Can you work these out from the model? Positions are in its coordinate system, mm. Round coordinates to 2 decimals unless told otherwise and drop trailing zeros. Order: outer loops, then holes, each group sorted by start corner. A loop starts at its lowest first (then second) coordinate and runs counter-clockwise, first axis right, second up.
Q1. We'd pull the mould along Z, two halves only. Please class faces 1 (the face through (-6.08, 76.021, 14.664)), 2 (the face through (4.468, 76.021, 14.188)): pulls with the +Z half, pulls with the -Z half, needs draft (parallel to the pull), parting line crosses it, or undercut.
Q2. If we section it at D-D (y = 73): Please give me the cut outline in (x, z) (3 decimals), plus the area to 3 significant figures.
Q3. If we section it at B-B (y = 11): Please give me the cut outline in (x, z) (3 decimals).
Q4. If we section it at C-C (x = 0): Please give me the cut outline in (y, z) (3 decimals).
Q5. If we section it at A-A (z = 0): Please give me the cut outline in (x, y) (3 decimals).
Q6. If I drill on line 1 (Z direction, x = -0.5, y = 8); line 2 (Z direction, x = -2.5, y = 72.5); line 3 (X direction, y = 122.5, z = 0) (3 decimals), over which ranges is the centre line in solid material (lowest first)?
Q7. Will these pins go through, and if not, where does the flat tip stop? P1, Ø1.5, axis at y = 59, z = -8, coming from the +X side; P2, Ø3, axis at x = 10, y = 22, coming from the +Z side; P3, Ø3, axis at x = 5.5, y = 68, coming from the +Z side.
from build123d import *

# Parameters (mm, degrees)
SKETCH1_R               = 15.875
SKETCH1_R_2             = 14.875
BOSS_EXTRUDE1_DEPTH     = 154.2
CUT_EXTRUDE1_DEPTH      = 154.2
CUT_EXTRUDE1_DEPTH_BACK = 154.2
SKETCH2_R               = 2.75


with BuildPart() as part:
    # Sketch1 → Boss-Extrude1 (new body)
    with BuildSketch(Plane(origin=(0, 0, 0), x_dir=(1, 0, 0), z_dir=(0, 1, 0))):
        with Locations(Location((0, 0, 0), (0, 0, 270))):
            Circle(SKETCH1_R)
        with Locations(Location((0, 0, 0), (0, 0, 270))):
            Circle(SKETCH1_R_2, mode=Mode.SUBTRACT)
    extrude(amount=BOSS_EXTRUDE1_DEPTH)

    # Sketch2 → Cut-Extrude1 (cut, two sides: drawn at the far end of the back side and taken through both)
    with BuildSketch(Plane.XY.offset(-CUT_EXTRUDE1_DEPTH_BACK)):
        with Locations(Location((-0.133461596, 143.2, 0), (0, 0, 180))):
            Circle(SKETCH2_R)
        with Locations(Location((-0.133461596, 11, 0), (0, 0, 180))):
            Circle(SKETCH2_R)
    extrude(amount=CUT_EXTRUDE1_DEPTH + CUT_EXTRUDE1_DEPTH_BACK, mode=Mode.SUBTRACT)


solid = part.part
Solution:
1. face 1: parting line crosses it
1. face 2: undercut
2. outline: circle Ø31.75 at (0, 0); hole circle Ø29.75 at (0, 0)
2. area: 96.6 mm2
3. outline: (-2.883, -15.611) - (-2.883, -14.593) arc R14.875 cw to (-2.883, 14.593) - (-2.883, 15.611) arc R15.875 ccw to start; (2.617, -15.658) arc R15.875 ccw to (2.617, 15.658) - (2.617, 14.643) arc R14.875 cw to (2.617, -14.643) - close
4. outline: (0, -15.875) - (8.253, -15.875) - (8.253, -14.875) - (0, -14.875) - close; (0, 14.875) - (8.253, 14.875) - (8.253, 15.875) - (0, 15.875) - close; (13.747, -15.875) - (140.453, -15.875) - (140.453, -14.875) - (13.747, -14.875) - close; (13.747, 14.875) - (140.453, 14.875) - (140.453, 15.875) - (13.747, 15.875) - close; (145.947, -15.875) - (154.2, -15.875) - (154.2, -14.875) - (145.947, -14.875) - close; (145.947, 14.875) - (154.2, 14.875) - (154.2, 15.875) - (145.947, 15.875) - close
5. outline: (-15.875, 0) - (-14.875, 0) - (-14.875, 154.2) - (-15.875, 154.2) - close; (14.875, 0) - (15.875, 0) - (15.875, 154.2) - (14.875, 154.2) - close
6. line 1: z = -15.87 to -14.87, 14.87 to 15.87
6. line 2: z = -15.68 to -14.66, 14.66 to 15.68
6. line 3: x = -15.875 to -14.875, 14.875 to 15.875
7. P1: stops at x = 14.12
7. P2: stops at z = 13.41
7. P3: stops at z = 15.36
